Geometry: final body of the model. Coordinates: model frame, mm. A direction names the side the tool comes from. Give positions to 0.01 mm unless a question says otherwise; leave off trailing zeros. Order: outer loops, then holes, each group sorted by start corner. A loop starts at its lowest first (then second) coordinate and runs counter-clockwise, first axis right, second up. Notation, with made-up numbers: (70.25, 86) - (125.25, 86) arc R27 ccw to (125.25, 124) - close; hole circle Ø6 at (-12.5, -16.5). An arc over 180 degrees is marked (long way). One line per item, written item: value.
```python
from build123d import *

# Parameters (mm, degrees)
F0_R     = 37.868067
F1_DEPTH = 45.974
F3_DEPTH = 25.4
F4_DEPTH = 20.575


with BuildPart() as f1:
    # F0 (on Top) → F1 (new body)
    with BuildSketch(Plane.XY):
        Circle(F0_R)
    extrude(amount=F1_DEPTH)

    # F2 (on face) → F3 (cut)
    with BuildSketch(Plane.XY.offset(45.974)):
        Polygon((6.691301, 20.593707), (-6.691301, 20.593707), (-17.518053, 12.727611), (-21.653504, 0), (-17.518053, -12.727611), (-6.691301, -20.593707), (6.691301, -20.593707), (17.518053, -12.727611), (21.653504, 0), (17.518053, 12.727611), align=None)
    extrude(amount=-F3_DEPTH, mode=Mode.SUBTRACT)

    # F3_face (on face) → F4 (cut, through all)
    with BuildSketch(Plane.XY.offset(20.574)):
        Polygon((21.653504, 0), (17.518053, 12.727611), (6.691301, 20.593707), (-6.691301, 20.593707), (-17.518053, 12.727611), (-21.653504, 0), (-17.518053, -12.727611), (-6.691301, -20.593707), (6.691301, -20.593707), (17.518053, -12.727611), align=None)
    extrude(amount=-F4_DEPTH, mode=Mode.SUBTRACT)


solid = f1.part
```
1) Section C-C, the plane y = -24. Return loops of the section in (x, z).
Answers below:
outline: (-29.29, 0) - (29.29, 0) - (29.29, 45.97) - (-29.29, 45.97) - close
2) Mould query, pull axis Y, two halves, no side actions, for faces 1 (the face through (-30.05, -23.04, 22.67)), 2 (the face through (16, -16, 0)), 3 (the face through (12.029, -16.716, 23.309)). Classes: released by +Y, released by -Y, zero draft, split by the parting line, or undercut.
Answers below:
face 1: split by the parting line
face 2: zero draft
face 3: undercut
3) Section D-D, the plane y = 27.5. Return loops of the section in (x, z).
Answers below:
outline: (-26.03, 0) - (26.03, 0) - (26.03, 45.97) - (-26.03, 45.97) - close
4) Material intervals for line 1 along X through (y, z) = (-15, 27.5); line 2 along X through (y, z) = (16, 13); line 3 along Y through (x, z) = (2, 7.5), sorted ascending.
Answers below:
line 1: -34.77 to -14.39, 14.39 to 34.77
line 2: -34.32 to -13.01, 13.01 to 34.32
line 3: -37.82 to -20.59, 20.59 to 37.82
5) Section B-B, the plane y = 9. Return loops of the section in (x, z).
Answers below:
outline: (-36.78, 0) - (-18.73, 0) - (-18.73, 45.97) - (-36.78, 45.97) - close; (18.73, 0) - (36.78, 0) - (36.78, 45.97) - (18.73, 45.97) - close
6) First-contact query: pin 1 (6 mm diameter, centred on x = 3, z = 33.5, fed in from +Y); pin 2 (5 mm diameter, centred on x = -6.5, z = 10.5, fed in from +Y); pin 3 (3 mm diameter, centred on y = -22, z = 18, fed in from -X). Flat tips, straight axial feed; report the tip coordinate or a pass-through.
Answers below:
pin 1: y = 37.87
pin 2: y = 37.66
pin 3: x = -31.84
7) Set-up query: faces 4 (the face through (0, -20.594, 23)), 5 (the face through (16, -16, 45.974)). Return all of +Z, -Z, +X, -X, +Y, -Y with unobstructed straight access to the full face (end or side cutting, diameter ignored); none if empty.
Answers below:
face 4: +Z, -Z
face 5: +Z, +X, -X, +Y, -Y
8) Section A-A, the plane x = 0. Return loops of the section in (y, z), then the cut area to 3 significant figures.
Answers below:
outline: (-37.87, 0) - (-20.59, 0) - (-20.59, 45.97) - (-37.87, 45.97) - close; (20.59, 0) - (37.87, 0) - (37.87, 45.97) - (20.59, 45.97) - close
area: 1,590 mm^2
